```python
from build123d import *

# Parameters (mm, degrees)
F0_W      = 42
F0_H      = 42
F1_DEPTH  = 10
F2_R      = 11
F3_DEPTH  = 2
F4_R      = 3.175
F6_DEPTH  = 12
F7_W      = 42
F7_H      = 42
F8_DEPTH  = 12
F9_R      = 5.08
F11_D     = 3
F11_DEPTH = 4
F11_TIP   = 0.9012909285
F12_R     = 2.5
F13_DEPTH = 22
F15_DEPTH = 2


with BuildPart() as f1:
    # F0 (on Top) → F1 (new body)
    with BuildSketch(Plane.XY):
        with Locations((0.959161669, -4.3165409938)):
            Rectangle(F0_W, F0_H)
    extrude(amount=F1_DEPTH)

    # F2 (on face) → F3 (join)
    with BuildSketch(Plane.XY.offset(10)):
        with Locations((0.959161669, -4.3165409938)):
            Circle(F2_R)
    extrude(amount=F3_DEPTH)

    # F4
    f4_edges = [f1.edges().sort_by_distance(p)[0] for p in [
        (21.959162, -25.316541, 5),
        (21.959162, 16.683459, 5),
        (-20.040838, 16.683459, 5),
        (-20.040838, -25.316541, 5),
    ]]
    fillet(f4_edges, radius=F4_R)

    # F5 (on face) → F6 (join)
    with BuildSketch(Plane(origin=(0, 0, 0), x_dir=(1, 0, 0), z_dir=(0, 0, -1))):
        Polygon((-20.040838331, 20.2365409938), (-20.040838331, -11.6034590062), (-14.960838331, -16.6834590062), (0.959161669, -16.6834590062), (16.879161669, -16.6834590062), (21.959161669, -11.6034590062), (21.959161669, 20.2365409938), (16.879161669, 25.3165409938), (0.959161669, 25.3165409938), (-14.960838331, 25.3165409938), align=None)
    extrude(amount=F6_DEPTH)

    # F7 (on face) → F8 (join)
    with BuildSketch(Plane(origin=(0, 0, -12), x_dir=(1, 0, 0), z_dir=(0, 0, -1))):
        with Locations((0.959161669, 4.3165409938)):
            Rectangle(F7_W, F7_H)
    extrude(amount=F8_DEPTH)

    # F9
    f9_edges = [f1.edges().sort_by_distance(p)[0] for p in [
        (21.959162, 16.683459, -18),
        (21.959162, -25.316541, -18),
        (-20.040838, 16.683459, -18),
        (-20.040838, -25.316541, -18),
    ]]
    fillet(f9_edges, radius=F9_R)

    # F11
    with Locations(Plane.XY.offset(10)):
        with Locations((-14.540838331, 11.1834590062), (-14.540838331, -19.8165409938), (16.459161669, -19.8165409938), (16.459161669, 11.1834590062)):
            Hole(F11_D / 2, depth=F11_DEPTH)
            with Locations((0, 0, -(F11_DEPTH + F11_TIP / 2))):  # 118° drill point
                Cone(0, F11_D / 2, F11_TIP, mode=Mode.SUBTRACT)

    # F12 (on face) → F13 (join)
    with BuildSketch(Plane.XY.offset(12)):
        with Locations((0.959161669, -4.3165409938)):
            Circle(F12_R)
    extrude(amount=F13_DEPTH)

    # F14 (on face) → F15 (join)
    with BuildSketch(Plane.XZ.offset(25.3165409938)):
        Polygon((-6.987169385, -24), (0.959161669, -24), (8.905492723, -24), (8.905492723, -20.8772607148), (0.959161669, -20.8772607148), (-6.987169385, -20.8772607148), align=None)
    extrude(amount=F15_DEPTH)


solid = f1.part
```
Work out the finished part from the listing and answer in its coordinate system (mm). A direction names the side the tool comes from. Coordinates: 2 decimals unless noted, no trailing zeros. Order: outer loops, then holes, each group sorted by start corner. A loop starts at its lowest first (then second) coordinate and runs counter-clockwise, first axis right, second up. Notation, with made-up numbers: M 31,6 L 68,6 A24 cw 68,20 Z; hole C -6.5,10.5 d3. An arc over 180 degrees is marked long. Use CSV: the item, a comma, the result in double quotes.
1) Consider line 1 (X direction, y = -18.5, z = 7); line 2 (Z direction, x = -4.5, y = -1.5); line 3 (Y direction, x = 8.5, z = -7). Determine where each line is inside the solid, lowest interval first. Write a range as [from, to].
Worked out:
line 1,"x = [-20.04, -15.26], [-13.82, 15.74], [17.18, 21.96]"
line 2,"z = [-24, 12]"
line 3,"y = [-25.32, 16.68]"
2) Determine the mould class of faces 5 (the face through (20.432, 15.235, -18.084)), 6 (the face through (20, 15, 0)), 7 (the face through (1, -26, -20.877)) for opening direction Z: released by +Z, released by -Z, zero draft, split by the parting line, or undercut.
Worked out:
face 5,"zero draft"
face 6,"undercut"
face 7,"released by +Z"
3) For faces 1 (the face through (-6.987, -26, -22)), 2 (the face through (17.958, -19.751, 7.972)), 3 (the face through (-17.47, -22.81, -5.92)), 4 (the face through (8.905, -26, -22)), determine the directions among +Z, -Z, +X, -X, +Y, -Y from which every point of the face is accessible in a straight line to the end or side of a thin tool.
Worked out:
face 1,"+Z, -Z, -X, -Y"
face 2,"+Z"
face 3,"-X, -Y"
face 4,"+Z, -Z, +X, -Y"
4) Section C-C on y = -23.5 is taken. Write down the section's boundary in (x, z).
Worked out:
outline,"M -19.74,0 L -16.78,0 L -16.78,-12 L -18.85,-12 L -18.85,-24 L 20.77,-24 L 20.77,-12 L 18.7,-12 L 18.7,0 L 21.65,0 L 21.65,10 L -19.74,10 Z"
5) Section D-D on x = 0 is taken. Write down the section's boundary in (y, z).
Worked out:
outline,"M -27.32,-24 L 16.68,-24 L 16.68,10 L 6.64,10 L 6.64,12 L -2.01,12 L -2.01,34 L -6.63,34 L -6.63,12 L -15.27,12 L -15.27,10 L -25.32,10 L -25.32,-20.88 L -27.32,-20.88 Z"
6) Section A-A on z = -16 is taken. Write down the section's boundary in (x, y), plus the area to 3 significant figures.
Worked out:
outline,"M -20.04,-20.24 A5.08 ccw -14.96,-25.32 L 16.88,-25.32 A5.08 ccw 21.96,-20.24 L 21.96,11.6 A5.08 ccw 16.88,16.68 L -14.96,16.68 A5.08 ccw -20.04,11.6 Z"
area,"1,740 mm^2"
7) Section B-B on x = -8 is taken. Write down the section's boundary in (y, z).
Worked out:
outline,"M -25.32,-24 L 16.68,-24 L 16.68,10 L 2.07,10 L 2.07,12 L -10.7,12 L -10.7,10 L -25.32,10 Z"
8) Flat-ended cylindrical pins translate along their axes: pin 1 Ø2 at (y, z) = (-26.5, -22.5) entering from +X; pin 2 Ø4 at (x, y) = (16, -19.5) entering from +Z; pin 3 Ø12.5 at (x, y) = (3.5, -14.5) entering from +Z. Find the tip coordinate at first contact, or state that the pin passes through.
Worked out:
pin 1,"stops at x = 8.91"
pin 2,"stops at z = 10"
pin 3,"stops at z = 12"
